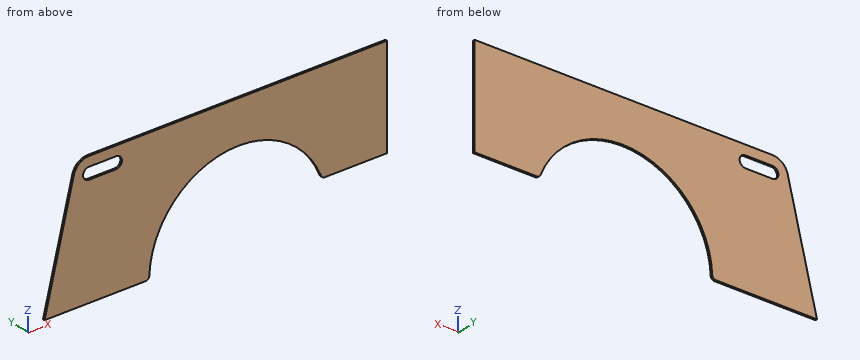
```python
from build123d import *

# Parameters (mm, degrees)
F1_DEPTH = 6.35


with BuildPart() as f1:
    # F0 (on Front) → F1 (new body)
    with BuildSketch(Plane.XZ):
        with BuildLine():
            Line((96.028596, 393.056471), (0, 0))
            Line((0, 0), (330.464698, 0))
            ThreePointArc((330.464698, 0), (339.255875, 3.534564), (343.153669, 12.170833))
            ThreePointArc((343.153669, 12.170833), (585.190634, 287.821884), (905.783947, 109.5375))
            ThreePointArc((905.783947, 109.5375), (910.457647, 103.769716), (917.557162, 101.6))
            Line((917.557162, 101.6), (1121.494123, 101.6))
            Line((1121.494123, 101.6), (1121.494123, 431.8))
            Line((1121.494123, 431.8), (145.377167, 431.8))
            ThreePointArc((145.377167, 431.8), (114.007028, 420.956906), (96.028596, 393.056471))
        make_face()
        with BuildLine():
            ThreePointArc((145.377167, 361.95), (126.327167, 381), (145.377167, 400.05))
            Line((145.377167, 400.05), (234.277167, 400.05))
            ThreePointArc((234.277167, 400.05), (253.327167, 381), (234.277167, 361.95))
            Line((234.277167, 361.95), (145.377167, 361.95))
        make_face(mode=Mode.SUBTRACT)
    extrude(amount=F1_DEPTH)


solid = f1.part
```
Model file for the job. Use its own axes, mm. Round coordinates to 2 decimals unless told otherwise and drop trailing zeros. Loops run counter-clockwise (first coordinate to the right, second up) from the corner with the lowest first, then second, coordinate; pieces in that order, holes last. Notation, with made-up numbers: M 84.5,-15 L 115.5,-15 A16 ccw 115.5,2 Z; hole C -1,15.5 d2. An arc over 180 degrees is marked long. Put each result on its own line as item: value. Start each with the question number.
Item 1: Cut at B-B (z = 273.5). List the corners of the cut face in (x, y).
Item 2: Drop flat-ended pins along their axis: P1, Ø3, axis at y = -3.5, z = 98, coming from the -X side; P2, Ø1, axis at x = 234, z = 205, coming from the +Y side. Give the stop position or say it passes through.
Item 3: Cut at A-A (y = -3.5). List the corners of the cut face in (x, z), then the cut area to 3 significant figures.
Item 4: Cut at C-C (x = 947.5). List the corners of the cut face in (y, z).
Item 5: Drill centre lines: line 1 along Z through (x, y) = (971.5, -1.75); line 2 along X through (y, z) = (-4, 266); line 3 along X through (y, z) = (-3, 113.5). Where is each one in solid material? Low to high.
Item 6: Cut at D-D (z = 196.5). List the corners of the cut face in (x, y).
Answer block:
1. outline: M 66.82,-6.35 L 532.43,-6.35 L 532.43,0 L 66.82,0 Z; M 737.57,-6.35 L 1121.49,-6.35 L 1121.49,0 L 737.57,0 Z
2. P1: x = 23.58
2. P2: y = 0
3. outline: M 0,0 L 330.46,0 A12.7 ccw 343.15,12.17 A292.1 cw 905.78,109.54 A12.7 ccw 917.56,101.6 L 1121.49,101.6 L 1121.49,431.8 L 145.38,431.8 A50.8 ccw 96.03,393.06 Z; hole M 145.38,361.95 L 234.28,361.95 A19.05 ccw 234.28,400.05 L 145.38,400.05 A19.05 ccw Z
3. area: 302,000 mm2
4. outline: M -6.35,101.6 L 0,101.6 L 0,431.8 L -6.35,431.8 Z
5. line 1: 101.6 to 431.8
5. line 2: 64.99 to 514.31, 755.69 to 1121.49
5. line 3: 27.73 to 365.85, 904.15 to 1121.49
6. outline: M 48.01,-6.35 L 418.87,-6.35 L 418.87,0 L 48.01,0 Z; M 851.13,-6.35 L 1121.49,-6.35 L 1121.49,0 L 851.13,0 Z
